Verification items for the finished model (mm, model axes). A direction names the side the tool comes from. Give positions to 0.01 mm unless a question says otherwise; leave off trailing zeros. Loops run counter-clockwise (first coordinate to the right, second up) from the corner with the lowest first, then second, coordinate; pieces in that order, holes last. Notation, with made-up numbers: (62.5, 81) -> (76.5, 81) arc R34 cw to (76.5, 111) -> close; hole circle Ø10 at (45.25, 17). An arc over 180 degrees is marked (long way). Answer in a Markdown table with one row per item. Add a question column.
Q1. Set-up check for faces 4 (the face through (0, 0, 10.2)), 5 (the face through (0, 1, 11.2)), 6 (the face through (0, -2, 4)): record each of +Z, -Z, +X, -X, +Y, -Y from which the full face is reachable in a straight line by a thin tool's end or side.
Q2. Gauge pin test, flat ends, axial feed: P1, Ø2, axis at y = -1.5, z = 9, coming from the +X side; P2, Ø1.1, axis at x = -0.5, y = 0, coming from the +Z side. Record the tip position at first contact, or that the pin passes through.
Q3. Section check B-B on y = 0. Enter the section's corners in (x, z).
Q4. Section check C-C on z = 2.5. Enter the section's corners in (x, y).
Q5. Section check A-A on x = 0. Enter the section's corners in (y, z).
Q6. Release check for a two-part mould opening along Y. For faces 1 (the face through (0, 0, 0)), 2 (the face through (0, -0.5, 11)), 3 (the face through (2.04, 0.64, 9.38)) record: pulls with the +Y half, pulls with the -Y half, needs draft (parallel to the pull), parting line crosses it, or undercut.
Q7. Section check D-D on z = 10. Enter the section's corners in (x, y).
Q8. Material ranges on probe 1 along Y at (x, z) = (-0.05, 6.25); probe 2 along Y at (x, z) = (2.25, 10.5); probe 3 along Z at (x, y) = (0.8, -0.15), recorded low to high.
```python
from build123d import *

# Parameters (mm, degrees)
BOX_W          = 10
BOX_H          = 1
BOX_DEPTH      = 1
CYLINDER_R     = 2
CYLINDER_DEPTH = 10


with BuildPart() as cub:
    # Box → Box (new body)
    with BuildSketch(Plane(origin=(-4, -0.5, 10.2), x_dir=(1, 0, 0), z_dir=(0, 0, 1))):
        with Locations((5, 0.5)):
            Rectangle(BOX_W, BOX_H)
    extrude(amount=BOX_DEPTH)


with BuildPart() as cut:
    # Cone → Cone (revolve)
    with BuildSketch(Plane(origin=(0, 0, 9), x_dir=(1, 0, 0), z_dir=(0, -1, 0))):
        Polygon((0, 0), (2, 0), (2.8, 2.2), (0, 2.2), align=None)
    revolve(axis=Axis((0, 0, 9), (0, 0, 1)))

    # Cut: cut Cub
    add(cub.part, mode=Mode.SUBTRACT)


with BuildPart() as obj1:
    # Cylinder → Cylinder (new body)
    with BuildSketch(Plane.XY):
        Circle(CYLINDER_R)
    extrude(amount=CYLINDER_DEPTH)

    # Fusion: union Cut
    add(cut.part)


solid = obj1.part
```
Taken from the geometry:
| question | item | result |
|---|---|---|
| 1 | face 4 | +Z, +X, -X |
| 1 | face 5 | +Z, +X, -X, +Y, -Y |
| 1 | face 6 | -Z |
| 2 | P1 | stops at x = 2.11 |
| 2 | P2 | stops at z = 11.2 |
| 3 | outline | (-2.44, 10.2) -> (-2, 9) -> (-2, 0) -> (2, 0) -> (2, 9) -> (2.44, 10.2) -> close |
| 4 | outline | circle Ø4 at (0, 0) |
| 5 | outline | (-2.8, 11.2) -> (-2, 9) -> (-2, 0) -> (2, 0) -> (2, 9) -> (2.8, 11.2) -> (0.5, 11.2) -> (0.5, 10.2) -> (-0.5, 10.2) -> (-0.5, 11.2) -> close |
| 6 | face 1 | needs draft |
| 6 | face 2 | undercut |
| 6 | face 3 | parting line crosses it |
| 7 | outline | circle Ø4.73 at (0, 0) |
| 8 | probe 1 | y = -2 to 2 |
| 8 | probe 2 | y = -1.19 to -0.5, 0.5 to 1.19 |
| 8 | probe 3 | z = 0 to 10.2 |
